For this review, take the finished solid that the model builds, in its own axes (mm). Face numbers are marked on the shaded views. A direction names the side the tool comes from. Give positions to 0.01 mm unless a question says otherwise; leave off trailing zeros. Write each loop counter-clockwise with the first axis right and the second up, starting at its lowest first coordinate (ties: lowest second). Pieces come first, ordered by that corner, then holes. Notation, with made-up numbers: M -6.75,-2.5 L 37.25,-2.5 A14 cw 37.25,16.5 Z; hole C -2.75,79 d2. An arc over 180 degrees is marked long. Write item = value, one per line.
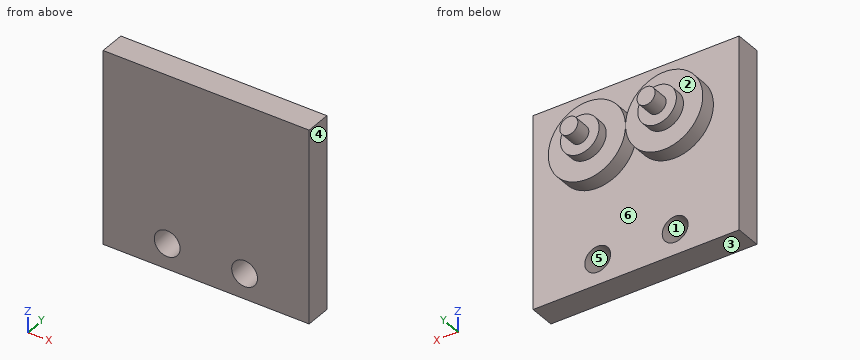
Autodesk Inventor part; units mm, degrees
ref_plane "YZ Plane" through (0, 0, 0) normal (1, 0, 0) x (0, 1, 0)
ref_plane "XZ Plane" through (0, 0, 0) normal (0, 1, 0) x (-1, 0, 0)
ref_plane "XY Plane" through (0, 0, 0) normal (0, 0, 1) x (1, 0, 0)
sketch "Sketch9" plane through (0, 0, 0) normal (0, 1, 0) x (-1, 0, 0)
  line L0 (0, 0) -> (127, 0)
  line L1 (127, 0) -> (127, -127)
  line L2 (127, -127) -> (0, -127)
  line L3 (0, -127) -> (0, 0)
  dimension "d29" = 127
  dimension "d30" = 127
extrude "Extrusion9" add sketch "Sketch9" along normal blind 12.7
sketch "Sketch10" plane through (0, 12.7, 0) normal (0, 1, 0) x (1, 0, 0)
  line L0 (-127, 127) -> (-127, 0)
  line L1 (-127, 0) -> (0, 0)
  line L2 (0, 0) -> (0, 127)
  line L3 (0, 127) -> (-127, 127)
  circle A0 centre (-89.0778, 50.9016) radius 19.0881
  circle A1 centre (-38.1762, 50.9016) radius 19.0881
  circle A2 centre (-82.7151, 101.8032) radius 6.3627
  circle A3 centre (-44.5389, 101.8032) radius 6.3627
  point P0 (-38.1762, 101.8032)
  dimension "d69" = 12.7254
  dimension "d70" = 12.7254
extrude "Extrusion10" cut sketch "Sketch10" against normal through all contours A2 | A3
sketch "Sketch11" plane through (0, 12.7, 0) normal (0, 1, 0) x (1, 0, 0)
  circle A0 centre (-82.55, 47.7782) radius 19.05
  circle A1 centre (-44.5389, 101.8032) radius 6.3627
  line L0 (-127, 0) -> (0, 0)
  circle A2 centre (-44.45, 47.7782) radius 19.05
  line L1 (-44.5389, 101.8032) -> (-44.5389, 95.4405)
  point P0 (-63.5, 47.7782)
  dimension "d47" = 38.1
  dimension "d48" = 38.1
extrude "Extrusion11" add sketch "Sketch11" along normal blind 7.62 contours A0 | A2
sketch "Sketch12" plane through (-127, 0, 0) normal (0, 0, 1) x (1, 0, 0)
  line L0 (0, 0) -> (0, 12.7)
  line L1 (127, 0) -> (0, 0)
  line L2 (0, 12.7) -> (127, 12.7)
  line L3 (127, 12.7) -> (127, 0)
  line L4 (127, 0) -> (0, 0)
  line L5 (0, 0) -> (0, 12.7)
extrude "Extrusion12" cut sketch "Sketch12" against normal blind 19.05
sketch "Sketch13" plane through (0, 0, -127) normal (0, 0, -1) x (-1, 0, 0)
  line L0 (0, 12.7) -> (127, 12.7)
  line L1 (127, 0) -> (127, 12.7)
  line L2 (0, 12.7) -> (127, 12.7)
  line L3 (127, 12.7) -> (127, 0)
  line L4 (127, 0) -> (0, 0)
  line L5 (0, 0) -> (0, 12.7)
extrude "Extrusion13" cut sketch "Sketch13" against normal blind 12.7
sketch "Sketch14" plane through (-127, 0, -19.05) normal (-1, 0, 0) x (0, 0, 1)
  line L0 (-95.25, 12.7) -> (0, 12.7)
  line L1 (-95.25, 0) -> (0, 0)
  line L2 (-95.25, 12.7) -> (0, 12.7)
  line L3 (0, 12.7) -> (0, 0)
  line L4 (0, 0) -> (-95.25, 0)
  line L5 (-95.25, 0) -> (-95.25, 12.7)
  point P0 (19.05, 0)
  point P1 (0, 12.7)
extrude "Extrusion14" cut sketch "Sketch14" against normal blind 12.7
sketch "Sketch15" plane through (0, 0, -19.05) normal (1, 0, 0) x (0, 0, -1)
  line L0 (0, 12.7) -> (0, 0)
  line L1 (95.25, 0) -> (95.25, 12.7)
  line L2 (0, 12.7) -> (95.25, 12.7)
  line L3 (95.25, 12.7) -> (95.25, 0)
  line L4 (95.25, 0) -> (0, 0)
  line L5 (0, 0) -> (0, 12.7)
  point P0 (-19.05, 0)
extrude "Extrusion15" cut sketch "Sketch15" against normal blind 12.7
sketch "Sketch16" plane through (-44.45, 20.32, -47.7782) normal (0, 1, 0) x (1, 0, 0)
  circle A0 centre (0, 0) radius 9.525
  point P0 (44.45, -47.7782)
  dimension "d59" = 19.05
extrude "Extrusion16" add sketch "Sketch16" along normal blind 5.08
sketch "Sketch17" plane through (-82.55, 20.32, -47.7782) normal (0, 1, 0) x (1, 0, 0)
  circle A0 centre (0, 0) radius 9.525
  point P0 (82.55, -47.7782)
  dimension "d62" = 19.05
extrude "Extrusion17" add sketch "Sketch17" along normal blind 5.08
sketch "Sketch18" plane through (-44.45, 25.4, -47.7782) normal (0, 1, 0) x (1, 0, 0)
  circle A0 centre (0, 0) radius 4.445
  circle A1 centre (-38.1, 0) radius 19.05
  circle A2 centre (-38.1, 0) radius 4.445
  point P0 (44.45, -47.7782)
  point P1 (-19.05, 0)
  dimension "d65" = 8.89
  dimension "d66" = 8.89
extrude "Extrusion18" add sketch "Sketch18" along normal blind 7.874 contours A0 | A2
sketch "Sketch19" plane through (0, 12.7, 0) normal (0, 1, 0) x (1, 0, 0)
  point P0 (0, 0)
sketch "Sketch20" plane through (0, 12.7, 0) normal (0, 1, 0) x (1, 0, 0)
  point P0 (0, 0)
sketch "Sketch21" plane through (-44.45, 33.274, -47.7782) normal (0, 1, 0) x (1, 0, 0)
  point P0 (44.45, -47.7782)
properties part number "Gripping Claws" material "Nickel-Copper Alloy 400"
1. We need section C-C, the plane z = -104. Write out the cut boundary in (x, y), then the cut area to 3 significant figures.
Responses:
outline = M -114.3,0 L -88.69,0 L -88.69,12.7 L -114.3,12.7 Z; M -76.74,0 L -50.51,0 L -50.51,12.7 L -76.74,12.7 Z; M -38.57,0 L -12.7,0 L -12.7,12.7 L -38.57,12.7 Z
area = 987 mm2
2. Machinability: for the marked faces 5 and 6, which of the approach directions +Z, -Z, +X, -X, +Y, -Y give a long, thin tool a straight path to every point of the face, cutting with its end or side? Answer none if there is none.
Responses:
face_5 = +Y, -Y
face_6 = +Y
3. For line 1 along Y through (x, z) = (-58.5, -105.5); line 2 along Y through (x, z) = (-54, -44); line 3 along Z through (x, y) = (-100, 18), list the stretches that pass through material, from the lowest coordinate up. Write a range as from..to.
Responses:
line_1 = 0..12.7
line_2 = 0..20.32
line_3 = -55.42..-40.14
4. We need section D-D, the plane y = 9.5. Write out the cut boundary in (x, z).
Responses:
outline = M -114.3,-114.3 L -12.7,-114.3 L -12.7,-19.05 L -114.3,-19.05 Z; hole C -82.72,-101.8 d12.73; hole C -44.54,-101.8 d12.73
5. We need section A-A, the plane x = -82.55. Write out the cut boundary in (y, z).
Responses:
outline = M 0,-114.3 L 12.7,-114.3 L 12.7,-108.16 L 0,-108.16 Z; M 0,-95.44 L 12.7,-95.44 L 12.7,-66.83 L 20.32,-66.83 L 20.32,-57.3 L 25.4,-57.3 L 25.4,-52.22 L 33.27,-52.22 L 33.27,-43.33 L 25.4,-43.33 L 25.4,-38.25 L 20.32,-38.25 L 20.32,-28.73 L 12.7,-28.73 L 12.7,-19.05 L 0,-19.05 Z
6. Insertion check: P1, Ø2, axis at x = -85.5, z = -69.5, coming from the -Y side; P2, Ø10, axis at x = -44.54, z = -101.8, coming from the +Y side; P3, Ø3, axis at y = 18, z = -62, coming from the -X side; P4, Ø12, axis at x = -32.5, y = 20, coming from the +Z side. Each pin has a flat end and moves straight along its axis. Give the tip position at first contact, or say it passes through.
Responses:
P1 = 0
P2 = through
P3 = -96.73
P4 = -29.68
7. The part is to be moulded in two halves that separate along X. For the marked faces 1, 2, 3 and 4, say which applies: +X half, -X half, draft (parallel to the pull), parting line (faces both ways), or undercut.
Responses:
face_1 = undercut
face_2 = undercut
face_3 = draft
face_4 = +X half
